Could you check a few things on this drawing? It's one solid part, dimensions in mm from its lowest x, y, z. Coordinates: 2 decimals unless noted, no trailing zeros. Write each loop counter-clockwise with the first axis right and the second up, starting at its lowest first coordinate (ties: lowest second). Pieces come first, ordered by that corner, then holes. Notation, with made-up numbers: (-16, -8) - (3, -8) arc R20 ccw to (3, 22) - close; hole circle Ø1 at (-11.75, 80). An arc over 180 degrees is marked (long way). Use one line per item in the form item = value. Start each with the question number.
(1) If we section it at C-C on y = 21.5: Please give me the cut outline in (x, z).
(2) If we section it at D-D on x = 4: Please give me the cut outline in (y, z).
(3) If we section it at A-A on z = 2.9: Please give me the cut outline in (x, y).
(4) Thinking about a two-plate mould opening in X: for the marked faces 1 and 2, which applies, pulls with the +X half, pulls with the -X half, needs draft (parallel to the pull), parting line crosses it, or undercut?
(5) If we section it at B-B on x = 46.5: Please give me the cut outline in (y, z), then the cut area to 3 significant figures.
(6) If I drill on probe 1 along Y at (x, z) = (40.5, 1.6); probe 2 along X at (y, z) = (16.5, 0.75); probe 3 along Y at (x, z) = (12.5, 2.35), over which ranges is the centre line in solid material (lowest first)? Write a range as from..to.
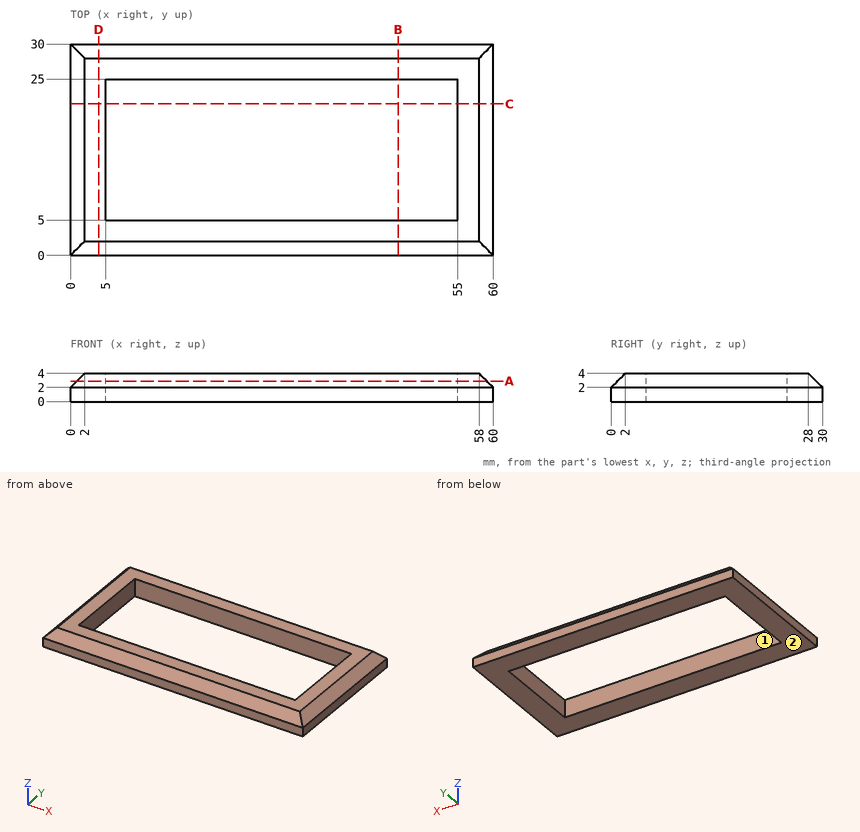
Reported:
q1.outline = (0, 0) - (5, 0) - (5, 4) - (2, 4) - (0, 2) - close; (55, 0) - (60, 0) - (60, 2) - (58, 4) - (55, 4) - close
q2.outline = (0, 0) - (30, 0) - (30, 2) - (28, 4) - (2, 4) - (0, 2) - close
q3.outline = (0.9, 0.9) - (59.1, 0.9) - (59.1, 29.1) - (0.9, 29.1) - close; hole (5, 5) - (55, 5) - (55, 25) - (5, 25) - close
q4.face_1 = undercut
q4.face_2 = needs draft
q5.outline = (0, 0) - (5, 0) - (5, 4) - (2, 4) - (0, 2) - close; (25, 0) - (30, 0) - (30, 2) - (28, 4) - (25, 4) - close
q5.area = 36.0 mm2
q6.probe_1 = 0..5, 25..30
q6.probe_2 = 0..5, 55..60
q6.probe_3 = 0.35..5, 25..29.65
